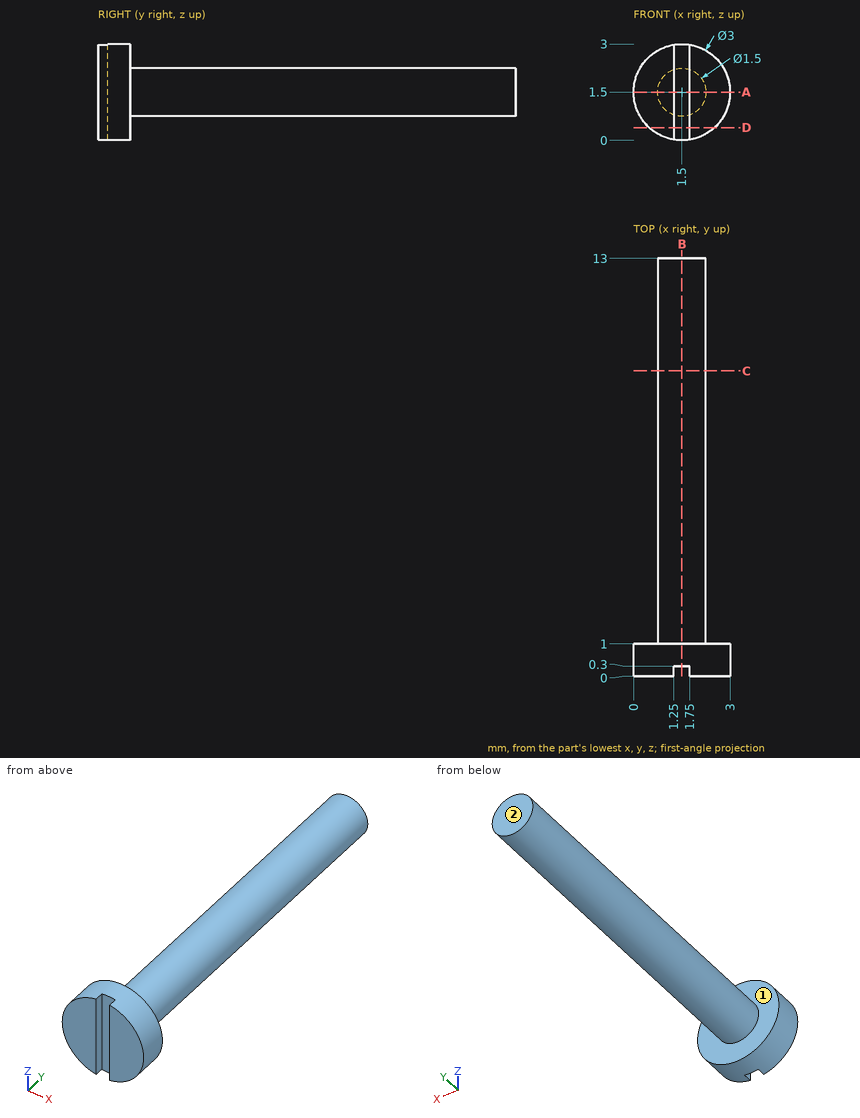
Study the drawing (mm; zero at the part's minimum x, y, z) and answer. A direction names the side the tool comes from. Round coordinates to 2 decimals unless told otherwise and drop trailing zeros. Write each loop counter-clockwise with the first axis right and the second up, starting at its lowest first coordinate (ties: lowest second). Pieces come first, ordered by that corner, then holes. Notation, with made-up numbers: (85.5, -30.5) -> (116.5, -30.5) arc R28 ccw to (116.5, -12.5) -> close; hole circle Ø5 at (58, 12). An arc over 180 degrees is marked (long way). Use CSV: the item, a comma, the result in double quotes. Start each with the question number.
(1) Each of these flat-tipped pins is pushed along its axis until it touches: pin 1 (1 mm diameter, centred on x = 0.5, y = 7, fed in from +Z); pin 2 (1 mm diameter, centred on y = 10.5, z = 2, fed in from +X). Where does it stop, or does it pass through?
(2) Section D-D on z = 0.4 is taken. Give the vertices of the cut face in (x, y), then the cut area to 3 significant figures.
(3) Which of the six approach directions +Z, -Z, +X, -X, +Y, -Y give full straight-line access (tool end or side, diameter ignored) to the marked faces 1 and 2?
(4) Section A-A on z = 1.5 is taken. Give the vertices of the cut face in (x, y), then the cut area to 4 significant figures.
(5) Consider L1, parallel to Y at x = 0.75, z = 0.7; L2, parallel to Y at x = 1.35, z = 1.1; L3, parallel to Z at x = 1.45, y = 3.5. Determine where each line is inside the solid, lowest interval first. Write a range as from..to.
(6) Section B-B on x = 1.5 is taken. Give the vertices of the cut face in (y, z).
(7) Section C-C on y = 9.5 is taken. Give the vertices of the cut face in (x, z), then the cut area to 3 significant figures.
A:
1,pin 1,"stops at z = 2.06"
1,pin 2,"stops at x = 2.25"
2,outline,"(0.48, 0) -> (1.25, 0) -> (1.25, 0.3) -> (1.75, 0.3) -> (1.75, 0) -> (2.52, 0) -> (2.52, 1) -> (0.48, 1) -> close"
2,area,"1.89 mm²"
3,face 1,"+Y"
3,face 2,"+Z, -Z, +X, -X, +Y"
4,outline,"(0, 0) -> (1.25, 0) -> (1.25, 0.3) -> (1.75, 0.3) -> (1.75, 0) -> (3, 0) -> (3, 1) -> (2.25, 1) -> (2.25, 13) -> (0.75, 13) -> (0.75, 1) -> (0, 1) -> close"
4,area,"20.85 mm²"
5,L1,"y = 0..1"
5,L2,"y = 0.3..13"
5,L3,"z = 0.75..2.25"
6,outline,"(0.3, 0) -> (1, 0) -> (1, 0.75) -> (13, 0.75) -> (13, 2.25) -> (1, 2.25) -> (1, 3) -> (0.3, 3) -> close"
7,outline,"circle Ø1.5 at (1.5, 1.5)"
7,area,"1.77 mm²"
